```python
from build123d import *

# Parameters (mm, degrees)
F0_W          = 1066.8
F0_H          = 609.6
F1_DEPTH      = 914.4
F2_W          = 1066.8
F2_H          = 50.8
F2_H_2        = 609.6
F3_DEPTH      = 50.8
F4_W          = 1066.8
F4_H          = 50.8
F5_DEPTH      = 152.4
F4_W_2        = 419.1
F4_H_2        = 419.1
F6_DEPTH      = 254
F7_R          = 76.2
F4_R          = 38.1
F8_DEPTH      = 228.6
F10_DEPTH     = 38.1
F11_T3_DEPTH  = 213.5462481737
F11_T6_DEPTH  = 213.5462481737
F11_T9_ANGLE  = 180
F11_T12_ANGLE = 180
F11_T15_ANGLE = 90
F11_T18_ANGLE = 90
F11_T21_ANGLE = 90
F11_T24_ANGLE = 90
F12_W         = 812.8
F12_H         = 355.6
F13_DEPTH     = 431.292
F14_W         = 1066.8
F14_H         = 71.1514726281
F15_DEPTH     = 50.8
F16_R         = 25.4
F17_DEPTH     = 25.4


# Not quite as in the source:
# - a fillet or chamfer that OpenCascade refuses, or shapes differently, is made with other operations: its cross-section is extruded or revolved along the edge and cut away or added


with BuildPart() as f1:
    # F0 (on Top) → F1 (new body)
    with BuildSketch(Plane.XY):
        Rectangle(F0_W, F0_H)
    extrude(amount=F1_DEPTH)

    # F2 (on face) → F3 (join)
    with BuildSketch(Plane.XY.offset(914.4)):
        with Locations((0, -330.2)):
            Rectangle(F2_W, F2_H)
        Rectangle(F2_W, F2_H_2)
    extrude(amount=-F3_DEPTH)

    # F4 (on face) → F5 (join)
    with BuildSketch(Plane.XY.offset(914.4)):
        with Locations((0, 279.4)):
            Rectangle(F4_W, F4_H)
    extrude(amount=F5_DEPTH)

    # F4 (on face) → F6 (cut)
    with BuildSketch(Plane.XY.offset(914.4)):
        with Locations((-247.65, -69.85)):
            Rectangle(F4_W_2, F4_H_2)
        with Locations((247.65, -69.85)):
            Rectangle(F4_W_2, F4_H_2)
    extrude(amount=-F6_DEPTH, mode=Mode.SUBTRACT)

    # F7
    f7_edges = [f1.edges().sort_by_distance(p)[0] for p in [
        (-247.65, 139.7, 660.4),
        (-457.2, -69.85, 660.4),
        (-247.65, -279.4, 660.4),
        (-38.1, -69.85, 660.4),
        (247.65, 139.7, 660.4),
        (38.1, -69.85, 660.4),
        (247.65, -279.4, 660.4),
        (457.2, -69.85, 660.4),
        (457.2, 139.7, 787.4),
        (38.1, 139.7, 787.4),
        (457.2, -279.4, 787.4),
        (38.1, -279.4, 787.4),
        (-457.2, -279.4, 787.4),
        (-38.1, -279.4, 787.4),
        (-38.1, 139.7, 787.4),
        (-457.2, 139.7, 787.4),
    ]]
    fillet(f7_edges, radius=F7_R)

    # F4 (on face) → F8 (join)
    with BuildSketch(Plane.XY.offset(914.4)):
        with Locations((0, 201.7975896597)):
            Circle(F4_R)
    extrude(amount=F8_DEPTH)

    # F9 (on Right) → F10 (join, symmetric)
    with BuildSketch(Plane.YZ):
        with BuildLine():
            Line((160.8298355818, 1219.2), (-52.7164125919, 1219.2))
            ThreePointArc((-52.7164125919, 1219.2), (-106.5979493183, 1196.8815367264), (-128.9164125919, 1143))
            ThreePointArc((-128.9164125919, 1143), (-97.7595895529, 1174.1568230391), (-66.6027665138, 1143))
            Line((-66.6027665138, 1143), (237.0298355818, 1143))
            ThreePointArc((237.0298355818, 1143), (214.7113723082, 1196.8815367264), (160.8298355818, 1219.2))
        make_face()
        with BuildLine():
            ThreePointArc((-66.6027665138, 1143), (-97.7595895529, 1174.1568230391), (-128.9164125919, 1143))
            Line((-128.9164125919, 1143), (-66.6027665138, 1143))
        make_face()
        with BuildLine():
            Line((-66.6027665138, 1143), (-128.9164125919, 1143))
            ThreePointArc((-128.9164125919, 1143), (-97.7595895529, 1111.8431769609), (-66.6027665138, 1143))
        make_face()
    extrude(amount=F10_DEPTH, both=True)

    # F11: fillet of radius 25.4 on 8 edges, made by hand


with BuildPart() as f11_tool1:
    # F11_s2 → F11_t3 (new body)
    with BuildSketch(Plane.XZ.offset(-160.8298355818)):
        with BuildLine():
            ThreePointArc((38.1, 1193.8), (30.6605122421, 1211.7605122421), (12.7, 1219.2))
            Line((12.7, 1219.2), (12.7, 1219.708))
            Line((12.7, 1219.708), (38.608, 1219.708))
            Line((38.608, 1219.708), (38.608, 1193.8))
            Line((38.608, 1193.8), (38.1, 1193.8))
        make_face()
    extrude(amount=F11_T3_DEPTH)


with BuildPart() as f11_tool4:
    # F11_s5 → F11_t6 (new body)
    with BuildSketch(Plane.XZ.offset(-160.8298355818)):
        with BuildLine():
            ThreePointArc((-38.1, 1193.8), (-30.6605122421, 1211.7605122421), (-12.7, 1219.2))
            Line((-12.7, 1219.2), (-12.7, 1219.708))
            Line((-12.7, 1219.708), (-38.608, 1219.708))
            Line((-38.608, 1219.708), (-38.608, 1193.8))
            Line((-38.608, 1193.8), (-38.1, 1193.8))
        make_face()
    extrude(amount=F11_T6_DEPTH)


with BuildPart() as f11_tool7:
    # F11_s8 → F11_t9 (revolve)
    with BuildSketch(Plane.XY.offset(1143)):
        with BuildLine():
            ThreePointArc((-12.7, -128.9164125919), (-30.6605122421, -121.4769248341), (-38.1, -103.5164125919))
            Line((-38.1, -103.5164125919), (-38.608, -103.5164125919))
            Line((-38.608, -103.5164125919), (-38.608, -129.4244125919))
            Line((-38.608, -129.4244125919), (-12.7, -129.4244125919))
            Line((-12.7, -129.4244125919), (-12.7, -128.9164125919))
        make_face()
    revolve(axis=Axis((-38.1, -97.7595895529, 1143), (1, 0, 0)), revolution_arc=F11_T9_ANGLE)


with BuildPart() as f11_tool10:
    # F11_s11 → F11_t12 (revolve)
    with BuildSketch(Plane.XY.offset(1143)):
        with BuildLine():
            ThreePointArc((12.7, -128.9164125919), (30.6605122421, -121.4769248341), (38.1, -103.5164125919))
            Line((38.1, -103.5164125919), (38.608, -103.5164125919))
            Line((38.608, -103.5164125919), (38.608, -129.4244125919))
            Line((38.608, -129.4244125919), (12.7, -129.4244125919))
            Line((12.7, -129.4244125919), (12.7, -128.9164125919))
        make_face()
    revolve(axis=Axis((38.1, -97.7595895529, 1143), (1, 0, 0)), revolution_arc=F11_T12_ANGLE)


with BuildPart() as f11_tool13:
    # F11_s14 → F11_t15 (revolve)
    with BuildSketch(Plane.XZ.offset(52.7164125919)):
        with BuildLine():
            ThreePointArc((38.1, 1193.8), (30.6605122421, 1211.7605122421), (12.7, 1219.2))
            Line((12.7, 1219.2), (12.7, 1219.708))
            Line((12.7, 1219.708), (38.608, 1219.708))
            Line((38.608, 1219.708), (38.608, 1193.8))
            Line((38.608, 1193.8), (38.1, 1193.8))
        make_face()
    revolve(axis=Axis((38.1, -52.7164125919, 1143), (1, 0, 0)), revolution_arc=F11_T15_ANGLE)


with BuildPart() as f11_tool16:
    # F11_s17 → F11_t18 (revolve)
    with BuildSketch(Plane.XY.offset(1143)):
        with BuildLine():
            ThreePointArc((38.1, 211.6298355818), (30.6605122421, 229.5903478239), (12.7, 237.0298355818))
            Line((12.7, 237.0298355818), (12.7, 237.5378355818))
            Line((12.7, 237.5378355818), (38.608, 237.5378355818))
            Line((38.608, 237.5378355818), (38.608, 211.6298355818))
            Line((38.608, 211.6298355818), (38.1, 211.6298355818))
        make_face()
    revolve(axis=Axis((38.1, 160.8298355818, 1143), (1, 0, 0)), revolution_arc=F11_T18_ANGLE)


with BuildPart() as f11_tool19:
    # F11_s20 → F11_t21 (revolve)
    with BuildSketch(Plane.XZ.offset(52.7164125919)):
        with BuildLine():
            ThreePointArc((-38.1, 1193.8), (-30.6605122421, 1211.7605122421), (-12.7, 1219.2))
            Line((-12.7, 1219.2), (-12.7, 1219.708))
            Line((-12.7, 1219.708), (-38.608, 1219.708))
            Line((-38.608, 1219.708), (-38.608, 1193.8))
            Line((-38.608, 1193.8), (-38.1, 1193.8))
        make_face()
    revolve(axis=Axis((-38.1, -52.7164125919, 1143), (1, 0, 0)), revolution_arc=F11_T21_ANGLE)


with BuildPart() as f11_tool22:
    # F11_s23 → F11_t24 (revolve)
    with BuildSketch(Plane.XY.offset(1143)):
        with BuildLine():
            ThreePointArc((-38.1, 211.6298355818), (-30.6605122421, 229.5903478239), (-12.7, 237.0298355818))
            Line((-12.7, 237.0298355818), (-12.7, 237.5378355818))
            Line((-12.7, 237.5378355818), (-38.608, 237.5378355818))
            Line((-38.608, 237.5378355818), (-38.608, 211.6298355818))
            Line((-38.608, 211.6298355818), (-38.1, 211.6298355818))
        make_face()
    revolve(axis=Axis((-38.1, 160.8298355818, 1143), (1, 0, 0)), revolution_arc=F11_T24_ANGLE)


with BuildPart() as f1_1:
    add(f1.part)

    # F11_t25: cut F11_tool1, F11_tool4, F11_tool7, F11_tool10, F11_tool13, F11_tool16, F11_tool19, F11_tool22
    add([f11_tool1.part, f11_tool4.part, f11_tool7.part, f11_tool10.part, f11_tool13.part, f11_tool16.part, f11_tool19.part, f11_tool22.part], mode=Mode.SUBTRACT)

    # F12 (on face) → F13 (cut)
    with BuildSketch(Plane(origin=(0, 0, 0), x_dir=(1, 0, 0), z_dir=(0, 0, -1))):
        Rectangle(F12_W, F12_H)
    extrude(amount=-F13_DEPTH, mode=Mode.SUBTRACT)

    # F14 (on face) → F15 (cut)
    with BuildSketch(Plane.XZ.offset(304.8)):
        with Locations((0, 35.5757363141)):
            Rectangle(F14_W, F14_H)
    extrude(amount=-F15_DEPTH, mode=Mode.SUBTRACT)

    # F16 (on face) → F17 (join)
    with BuildSketch(Plane.XZ.offset(304.8)):
        with Locations((-116.0961332864, 698.1492042542)):
            Circle(F16_R)
        with Locations((91.3885235786, 698.1492042542)):
            Circle(F16_R)
    extrude(amount=F17_DEPTH)


solid = f1_1.part
```
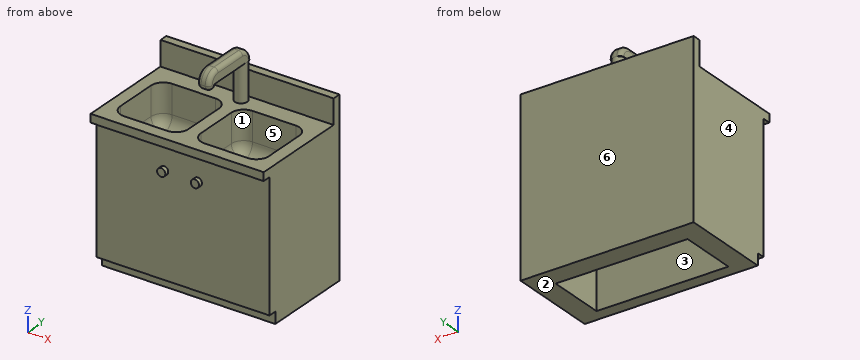
Input: part model. Units: mm. Frame: model coordinates. Face numbers are marked on the shaded views. A direction names the side the tool comes from. Give positions to 0.01 mm unless a question says otherwise; leave off trailing zeros. Order: outer loops, then holes, each group sorted by start corner. A loop starts at its lowest first (then second) coordinate and runs counter-clockwise, first axis right, second up.
1. Cut plane C-C (z = 395). Return loops of the section in (x, y).
Computed:
outline: (-533.4, -304.8) - (533.4, -304.8) - (533.4, 304.8) - (-533.4, 304.8) - close; hole (-406.4, -177.8) - (406.4, -177.8) - (406.4, 177.8) - (-406.4, 177.8) - close
2. Line query: probe 1 along X at (y, z) = (-172, 823); probe 2 along Y at (x, z) = (-167, 834); probe 3 along X at (y, z) = (75.5, 70). Output: solid intervals per line, ascending.
Computed:
probe 1: x = -533.4 to -457.2, -38.1 to 38.1, 457.2 to 533.4
probe 2: y = -304.8 to -279.4, 139.7 to 304.8
probe 3: x = -533.4 to -406.4, 406.4 to 533.4
3. Cut plane B-B (y = -30). Return loops of the section in (x, z), and give its area (3 significant figures).
Computed:
outline: (-533.4, 0) - (-406.4, 0) - (-406.4, 431.29) - (406.4, 431.29) - (406.4, 0) - (533.4, 0) - (533.4, 914.4) - (457.2, 914.4) - (457.2, 736.6) arc R76.2 cw to (381, 660.4) - (114.3, 660.4) arc R76.2 cw to (38.1, 736.6) - (38.1, 914.4) - (-38.1, 914.4) - (-38.1, 736.6) arc R76.2 cw to (-114.3, 660.4) - (-381, 660.4) arc R76.2 cw to (-457.2, 736.6) - (-457.2, 914.4) - (-533.4, 914.4) - close; (-38.1, 1143) - (38.1, 1143) - (38.1, 1193.8) arc R25.4 ccw to (12.7, 1219.2) - (-12.7, 1219.2) arc R25.4 ccw to (-38.1, 1193.8) - close
area: 423,000 mm2
4. Cut plane D-D (z = 840). Return loops of the section in (x, y), and give its area (3 significant figures).
Computed:
outline: (-533.4, -304.8) - (533.4, -304.8) - (533.4, 304.8) - (-533.4, 304.8) - close; hole (-457.2, -203.2) arc R76.2 ccw to (-381, -279.4) - (-114.3, -279.4) arc R76.2 ccw to (-38.1, -203.2) - (-38.1, 63.5) arc R76.2 ccw to (-114.3, 139.7) - (-381, 139.7) arc R76.2 ccw to (-457.2, 63.5) - close; hole (38.1, -203.2) arc R76.2 ccw to (114.3, -279.4) - (381, -279.4) arc R76.2 ccw to (457.2, -203.2) - (457.2, 63.5) arc R76.2 ccw to (381, 139.7) - (114.3, 139.7) arc R76.2 ccw to (38.1, 63.5) - close
area: 309,000 mm2
5. Pin query (flat end, axial travel): pin 1 Ø2 at (x, y) = (345.5, 67.5) entering from -Z; pin 2 Ø1.5 at (x, y) = (-89.5, -145.5) entering from +Z; pin 3 Ø4 at (x, y) = (-235, -93) entering from +Z. Return the tip coordinate at first contact, or that it passes through.
Computed:
pin 1: stops at z = 431.29
pin 2: stops at z = 664.81
pin 3: stops at z = 660.4
6. Set-up query: the marked faces 1, 2 and 3. Return all of +Z, -Z, +X, -X, +Y, -Y with unobstructed straight access to the full face (end or side cutting, diameter ignored); none if empty.
Computed:
face 1: +Z
face 2: -Z, +X, -X, +Y, -Y
face 3: -Z
7. Draft query along Y for the marked faces 4, 5 and 6. Return one class per face: released by +Y, released by -Y, zero draft, split by the parting line, or undercut.
Computed:
face 4: zero draft
face 5: undercut
face 6: released by +Y
8. Cut plane A-A (z = 965.5). Return loops of the section in (x, y), and give its area (3 significant figures).
Computed:
outline: (-533.4, 254) - (533.4, 254) - (533.4, 304.8) - (-533.4, 304.8) - close; circle Ø76.2 at (0, 201.8)
area: 58,800 mm2
